Here's how the part is built. I have some questions about the finished solid (model axes, mm). A direction names the side the tool comes from. Coordinates: 2 decimals unless noted, no trailing zeros. Write each loop counter-clockwise with the first axis right and the second up, starting at its lowest first coordinate (ties: lowest second). Pieces come first, ordered by that corner, then holes.
(1) Which directions (+Z, -Z, +X, -X, +Y, -Y) give clear straight access to the entire face, cutting with the end or side of a thin tool? Please do faces 3 (the cylindrical face through (8.52, -20.35, 2.43)), 4 (the cylindrical face through (6.923, -3.726, -3.124)), 5 (the cylindrical face through (2.465, 7.91, -10.316)).
(2) Please list where these lines run through material, in increasing order: probe 1 along Z at (x, y) = (8.5, -3.5); probe 2 along Y at (x, z) = (3.6, 0); probe 3 along X at (y, z) = (-1.5, 7.5).
(3) Imagine slicing it at D-D, the plane y = -12. List the corners of the cut face in (x, z) for me.
(4) Thinking about a two-plate mould opening in Y: for faces 1 (the cylindrical face through (5.07, 15.821, -20.633)), 2 (the cylindrical face through (8.52, -2.43, -20.35)), which applies, released by +Y, released by -Y, zero draft, split by the parting line, or undercut?
(5) Imagine slicing it at B-B, the plane x = 1.5. List the corners of the cut face in (y, z) for me, plus the area to 3 significant figures.
(6) For pin 1 Ø3.5 at (y, z) = (19.29, -2.87) entering from +X; pin 2 Ø1.8 at (y, z) = (-4.8, -3.36) entering from +X; pin 3 Ø1.5 at (y, z) = (9.5, -6) entering from -X; pin 4 Ø1.4 at (y, z) = (-19.29, 2.87) entering from +X, each with a flat end and sliding along its axis, tell me the tip position at first contact or that it passes through.
(7) Imagine slicing it at C-C, the plane z = -9.5. List the corners of the cut face in (x, y) for me, plus the area to 3 significant figures.
(8) Imagine slicing it at A-A, the plane y = 0. List the corners of the cut face in (x, z) for me.
```python
from build123d import *

# Parameters (mm, degrees)
HOLE_WIZARD_M22_D           = 2.2
HOLE_WIZARD_M22_CSINK_D     = 4.4
HOLE_WIZARD_M22_CSINK_ANGLE = 90
PATTERN_CIRCULAR_2_COUNT    = 4
PATTERN_CIRCULAR_3_COUNT    = 4


with BuildPart() as part:
    # Sketch 1 → Revolve 1 (revolve)
    with BuildSketch(Plane.XY, mode=Mode.PRIVATE) as revolve_1_sk:
        Polygon((0, 13), (0, 26), (10, 26), (10, 2.6), (5, 2.6), (5, 13), align=None)
    revolve(revolve_1_sk.sketch.rotate(Axis((0, 0, 0), (1, 0, 0)), 90), axis=Axis((0, 0, 0), (1, 0, 0)))

    # Hole Wizard M22 (through all)
    with Locations(Plane(origin=(10, 0, 0), x_dir=(0, 0, -1), z_dir=(1, 0, 0))):
        with Locations((-3.362654925, 4.8)):
            hole_wizard_m22 = CounterSinkHole(HOLE_WIZARD_M22_D / 2, HOLE_WIZARD_M22_CSINK_D / 2, counter_sink_angle=HOLE_WIZARD_M22_CSINK_ANGLE)

    # Pattern Circular 2: Hole Wizard M22 ×4 about axis
    pattern_circular_2_axis = Axis((0, 0, 0), (1, 0, 0))
    for i in range(1, PATTERN_CIRCULAR_2_COUNT):
        add(hole_wizard_m22.rotate(pattern_circular_2_axis, i * 360 / PATTERN_CIRCULAR_2_COUNT), mode=Mode.SUBTRACT)

    # Sketch 7 → Hole Wizard M2.21 (revolve, cut)
    with BuildSketch(Plane(origin=(10, -2.866446976, -19.288169476), x_dir=(0, 0, -1), z_dir=(0, 1, 0))):
        Polygon((0, 0), (0, 3.690989712), (1.15, 3), (1.15, 0), align=None)
    hole_wizard_m2_21 = revolve(axis=Axis((16.35, -2.866446976, -19.288169476), (-1, 0, 0)), mode=Mode.SUBTRACT)

    # Pattern Circular 3: Hole Wizard M2.21 ×4 about axis
    pattern_circular_3_axis = Axis((0, 0, 0), (1, 0, 0))
    for i in range(1, PATTERN_CIRCULAR_3_COUNT):
        add(hole_wizard_m2_21.rotate(pattern_circular_3_axis, i * 360 / PATTERN_CIRCULAR_3_COUNT), mode=Mode.SUBTRACT)


solid = part.part
```
Recorded:
1. face 3: +X
1. face 4: +X, -X
1. face 5: -X
2. probe 1: z = -25.76 to -20.25, -18.33 to 3.71, 5.89 to 25.76
2. probe 2: y = -26 to -13, 13 to 26
2. probe 3: x = 5 to 10
3. outline: (0, -23.07) - (10, -23.07) - (10, 23.07) - (0, 23.07) - (0, 5) - (5, 5) - (5, -5) - (0, -5) - close
4. face 1: split by the parting line
4. face 2: undercut
5. outline: circle Ø52 at (0, 0); hole circle Ø26 at (0, 0)
5. area: 1,590 mm2
6. pin 1: stops at x = 10
6. pin 2: passes through
6. pin 3: stops at x = 5
6. pin 4: stops at x = 6.73
7. outline: (0, -24.2) - (10, -24.2) - (10, 24.2) - (0, 24.2) - (0, 8.87) - (5, 8.87) - (5, -8.87) - (0, -8.87) - close
7. area: 395 mm2
8. outline: (0, -26) - (10, -26) - (10, -2.6) - (5, -2.6) - (5, -13) - (0, -13) - close; (0, 13) - (5, 13) - (5, 2.6) - (10, 2.6) - (10, 26) - (0, 26) - close
